Design review of the part built by this model. Coordinates are the model's own, in mm. Face numbers are marked on the shaded views. A direction names the side the tool comes from. Coordinates: 2 decimals unless noted, no trailing zeros. Loops run counter-clockwise (first coordinate to the right, second up) from the corner with the lowest first, then second, coordinate; pieces in that order, holes last. Notation, with made-up numbers: (43, 83.5) - (93, 83.5) arc R24 ccw to (93, 102.5) - close; hole circle Ø11 at (-34, -0.5). An arc over 180 degrees is marked (long way). Return JSON: item names as keys, results as strings. Group by question number.
from build123d import *

# Parameters (mm, degrees)
BOSS_EXTRUDE1_DEPTH      = 50
SKETCH2_OUTSIDE_W        = 130.372
SKETCH2_OUTSIDE_H        = 120.372
SKETCH2_OUTSIDE_R        = 5
SKETCH2_OUTSIDE_R_2      = 3.25
CUT_EXTRUDE34_DEPTH      = 46
CUT_EXTRUDE34_DEPTH_BACK = 1
BOSS_EXTRUDE3_DEPTH      = 4.5
FILLET3_R                = 2.5
FILLET4_R                = 7
SKETCH6_R                = 3.25
CUT_EXTRUDE35_DEPTH      = 1
CUT_EXTRUDE35_DEPTH_BACK = 88.5
CUT_EXTRUDE39_DEPTH      = 3.18


with BuildPart() as part:
    # Sketch1 → Boss-Extrude1 (new body, symmetric)
    with BuildSketch(Plane(origin=(0, 0, 0), x_dir=(0, 0, -1), z_dir=(1, 0, 0))):
        Polygon((0, 0), (0, 45), (4.5, 45), (4.5, 4.5), (90, 4.5), (90, 0), align=None)
    extrude(amount=BOSS_EXTRUDE1_DEPTH, both=True)

    # Sketch2 outside → Cut-Extrude34 (cut, two sides)
    with BuildSketch(Plane(origin=(0, 0, 0), x_dir=(1, 0, 0), z_dir=(0, 1, 0))) as cut_extrude34_sk:
        with Locations((0, 45)):
            Rectangle(SKETCH2_OUTSIDE_W, SKETCH2_OUTSIDE_H)
        with BuildLine():
            Line((-40, 45), (-25.836010131, 45))
            ThreePointArc((-25.836010131, 45), (-17.535836731, 41.561955607), (-14.097792338, 33.261782207))
            Line((-14.097792338, 33.261782207), (-14.097792338, 7))
            Line((-14.097792338, 7), (13.661782207, 7))
            Line((13.661782207, 7), (13.661782207, 33.261782207))
            ThreePointArc((13.661782207, 33.261782207), (17.099826599, 41.561955607), (25.4, 45))
            Line((25.4, 45), (40, 45))
            ThreePointArc((40, 45), (47.071067812, 47.928932188), (50, 55))
            Line((50, 55), (50, 80))
            ThreePointArc((50, 80), (47.071067812, 87.071067812), (40, 90))
            Line((40, 90), (-40, 90))
            ThreePointArc((-40, 90), (-47.071067812, 87.071067812), (-50, 80))
            Line((-50, 80), (-50, 55))
            ThreePointArc((-50, 55), (-47.071067812, 47.928932188), (-40, 45))
        make_face(mode=Mode.SUBTRACT)
        with Locations((-25, 67.5)):
            Circle(SKETCH2_OUTSIDE_R)
        with Locations((25, 67.5)):
            Circle(SKETCH2_OUTSIDE_R)
        with Locations((25, 81.04)):
            Circle(SKETCH2_OUTSIDE_R_2)
        with Locations((25, 53.96)):
            Circle(SKETCH2_OUTSIDE_R_2)
        with Locations((38.54, 67.5)):
            Circle(SKETCH2_OUTSIDE_R_2)
        with Locations((-25, 81.04)):
            Circle(SKETCH2_OUTSIDE_R_2)
        with Locations((-25, 53.96)):
            Circle(SKETCH2_OUTSIDE_R_2)
        with Locations((-38.54, 67.5)):
            Circle(SKETCH2_OUTSIDE_R_2)
        Polygon((-2.5, 79.24), (2.5, 79.24), (7.5, 74.24), (7.5, 60.76), (2.5, 55.76), (-2.5, 55.76), (-7.5, 60.76), (-7.5, 74.24), align=None)
    extrude(amount=CUT_EXTRUDE34_DEPTH, mode=Mode.SUBTRACT)
    extrude(cut_extrude34_sk.sketch, amount=-CUT_EXTRUDE34_DEPTH_BACK, mode=Mode.SUBTRACT)

    # Sketch4 → Boss-Extrude3 (add)
    with BuildSketch(Plane.XY.offset(-7)):
        with BuildLine():
            Line((-14.097792338, 0), (-14.097792338, 45))
            ThreePointArc((-14.097792338, 45), (-13.365559291, 46.767766953), (-11.597792338, 47.5))
            Line((-11.597792338, 47.5), (13.661782207, 47.5))
            Line((13.661782207, 47.5), (21.222778521, 43.209368433))
            Line((21.222778521, 43.209368433), (21.222778521, 21.944029683))
            Line((21.222778521, 21.944029683), (13.661782207, 17.653398116))
            Line((13.661782207, 17.653398116), (13.661782207, 4.5))
            Line((13.661782207, 4.5), (13.661782207, 0))
            Line((13.661782207, 0), (-14.097792338, 0))
        make_face()
    extrude(amount=BOSS_EXTRUDE3_DEPTH)

    # Fillet3
    fillet3_edges = [part.edges().sort_by_distance(p)[0] for p in [
        (-0.218005066, 4.5, -7),
    ]]
    fillet(fillet3_edges, radius=FILLET3_R)

    # Fillet4
    fillet4_edges = [part.edges().sort_by_distance(p)[0] for p in [
        (-0.218005066, 0, -2.5),
    ]]
    fillet(fillet4_edges, radius=FILLET4_R)

    # Sketch6 → Cut-Extrude35 (cut, two sides)
    with BuildSketch(Plane.XY.offset(-2.5)) as cut_extrude35_sk:
        with Locations((-0.297792338, 40.083077312)):
            Circle(SKETCH6_R)
        with Locations((-0.297792338, 25.083077312)):
            Circle(SKETCH6_R)
    extrude(amount=CUT_EXTRUDE35_DEPTH, mode=Mode.SUBTRACT)
    extrude(cut_extrude35_sk.sketch, amount=-CUT_EXTRUDE35_DEPTH_BACK, mode=Mode.SUBTRACT)

    # Sketch7 → Cut-Extrude39 (cut)
    with BuildSketch(Plane.XY.offset(-2.5)):
        with BuildLine():
            Line((18.539617084, 41.355633115), (18.539617084, 36.032215871))
            ThreePointArc((18.539617084, 36.032215871), (16.149617084, 33.642215871), (13.759617084, 36.032215871))
            Line((13.759617084, 36.032215871), (13.759617084, 41.355633115))
            ThreePointArc((13.759617084, 41.355633115), (16.149617084, 43.745633115), (18.539617084, 41.355633115))
        make_face()
        with BuildLine():
            Line((18.539617084, 28.355633115), (18.539617084, 23.032215871))
            ThreePointArc((18.539617084, 23.032215871), (16.149617084, 20.642215871), (13.759617084, 23.032215871))
            Line((13.759617084, 23.032215871), (13.759617084, 28.355633115))
            ThreePointArc((13.759617084, 28.355633115), (16.149617084, 30.745633115), (18.539617084, 28.355633115))
        make_face()
    extrude(amount=-CUT_EXTRUDE39_DEPTH, mode=Mode.SUBTRACT)


solid = part.part
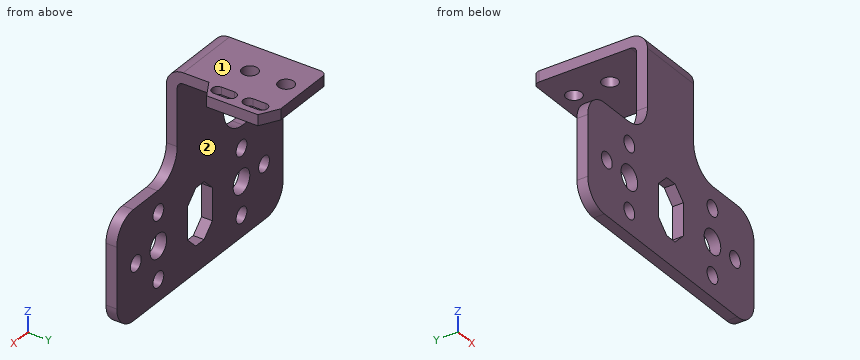
Item 1: To check wall thickness, follow line 1 (X direction, y = 1.6, z = -67.5); line 2 (Z direction, x = 25, y = 2); line 3 (X direction, y = 2.2, z = -53.96). State the ranges of each line that lie inside material, in increasing order. Write a range as from..to.
Item 2: For the marked faces 1 and 2, list the 3-axis set-ups (+Z, -Z, +X, -X, +Y, -Y) from which the entire face can be reached by the end or side of a thin tool; tool diameter is ignored.
Item 3: Add section B-B (z = -67.5). State the section outline as (x, y) points, then the cut area to 3 significant figures.
Item 4: Add section A-A (x = 38.54). State the section outline as (y, z) points, then the cut area to 3 significant figures.
Item 5: Add section C-C (z = -20). State the section outline as (x, y) points, then the cut area to 3 significant figures.
Item 6: For P1, Ø1, axis at x = 2, z = -46, coming from the +Y side; P2, Ø3.5, axis at y = 39, z = -4.5, coming from the -X side; P3, Ø12, axis at x = 3.5, y = 34, coming from the -Z side, all flat-tipped, find the tip position at first contact; note any pin that passes through.
Answers below:
{
 "1": {"line 1": "x = -50..-41.79, -35.29..-30, -20..-7.5, 7.5..20, 30..35.29, 41.79..50", "line 2": "z = -90..-84.29, -77.79..-72.5, -62.5..-57.21, -50.71..-44.99", "line 3": "x = -49.95..-28.25, -21.75..21.75, 28.25..49.95"},
 "2": {"face 1": "+Z, +X, -X, +Y, -Y", "face 2": "-Z, +X, -X, +Y"},
 "3": {"outline": "(-50, 0) - (-41.79, 0) - (-41.79, 4.5) - (-50, 4.5) - close; (-35.29, 0) - (-30, 0) - (-30, 4.5) - (-35.29, 4.5) - close; (-20, 0) - (-7.5, 0) - (-7.5, 4.5) - (-20, 4.5) - close; (7.5, 0) - (20, 0) - (20, 4.5) - (7.5, 4.5) - close; (30, 0) - (35.29, 0) - (35.29, 4.5) - (30, 4.5) - close; (41.79, 0) - (50, 0) - (50, 4.5) - (41.79, 4.5) - close", "area": "234 mm^2"},
 "4": {"outline": "(0, -90) - (4.5, -90) - (4.5, -70.75) - (0, -70.75) - close; (0, -64.25) - (4.5, -64.25) - (4.5, -45) - (0, -45) - close", "area": "173 mm^2"},
 "5": {"outline": "(-14.1, 0) - (13.66, 0) - (13.66, 4.5) - (-14.1, 4.5) - close", "area": "125 mm^2"},
 "6": {"P1": "stops at y = 4.5", "P2": "stops at x = -14.1", "P3": "stops at z = -7"}
}
